```python
from build123d import *

# Parameters (mm, degrees)
SKETCH_1_W      = 48
SKETCH_1_H      = 80
SKETCH_1_R      = 1.55
EXTRUDE_1_DEPTH = 1.5


with BuildPart() as part:
    # 草图1 → 凸台-拉伸1 (new body)
    with BuildSketch(Plane(origin=(0, 0, 0), x_dir=(1, 0, 0), z_dir=(0, 1, 0))):
        Rectangle(SKETCH_1_W, SKETCH_1_H)
        with Locations(Location((-22, 22, 0), (0, 0, 270))):
            Circle(SKETCH_1_R, mode=Mode.SUBTRACT)
        with Locations(Location((22, 22, 0), (0, 0, 90))):
            Circle(SKETCH_1_R, mode=Mode.SUBTRACT)
        with Locations(Location((22, -22, 0), (0, 0, 270))):
            Circle(SKETCH_1_R, mode=Mode.SUBTRACT)
        with Locations(Location((-22, -22, 0), (0, 0, 90))):
            Circle(SKETCH_1_R, mode=Mode.SUBTRACT)
        Polygon((22.62, 35), (21.62, 34), (20.62, 35), (21.62, 36), align=None, mode=Mode.SUBTRACT)
        Polygon((-21.62, 34), (-20.62, 35), (-21.62, 36), (-22.62, 35), align=None, mode=Mode.SUBTRACT)
        Polygon((21.62, -36), (22.62, -35), (21.62, -34), (20.62, -35), align=None, mode=Mode.SUBTRACT)
        Polygon((-22.62, -35), (-21.62, -34), (-20.62, -35), (-21.62, -36), align=None, mode=Mode.SUBTRACT)
    extrude(amount=EXTRUDE_1_DEPTH)


solid = part.part
```
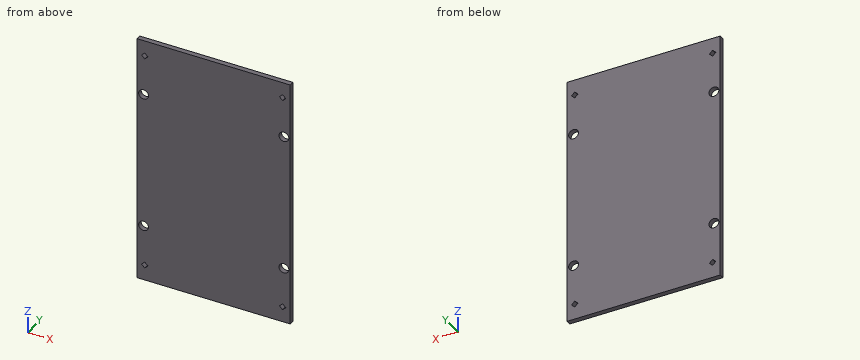
Could you check a few things on this model? Use its own coordinates, in mm. Round coordinates to 2 decimals unless told otherwise and drop trailing zeros. Write each loop counter-clockwise with the first axis right and the second up, starting at its lowest first coordinate (ties: lowest second). Pieces come first, ordered by that corner, then holes. Notation, with made-up numbers: M 6.5,69 L 33.5,69 A20 cw 33.5,73 Z; hole C 17.25,78.25 d11. An arc over 180 degrees is marked long. Answer in a Markdown table with one row per item. Add a question column.
Q1. Will this pin go through, and if not, where does the flat tip stop? pin 1 Ø3 at (x, z) = (-22, -22) entering from +Y.
Q2. If I drill on line 1 (X direction, y = 0.5, z = -22); line 2 (X direction, y = 0.8, z = -35), over which ranges is the centre line in solid material (lowest first)? Write a range as from..to.
Q3. Imagine slicing it at A-A (z = 22). Please give me the cut outline in (x, y), then the cut area to 3 significant figures.
Values:
| question | item | result |
|---|---|---|
| 1 | pin 1 | through |
| 2 | line 1 | -24..-23.55, -20.45..20.45, 23.55..24 |
| 2 | line 2 | -24..-22.62, -20.62..20.62, 22.62..24 |
| 3 | outline | M -24,0 L -23.55,0 L -23.55,1.5 L -24,1.5 Z; M -20.45,0 L 20.45,0 L 20.45,1.5 L -20.45,1.5 Z; M 23.55,0 L 24,0 L 24,1.5 L 23.55,1.5 Z |
| 3 | area | 62.7 mm^2 |
